Read the model definition and answer for the solid it produces. Units are mm, in the model's axes. Round coordinates to 2 decimals unless told otherwise and drop trailing zeros. Order: outer loops, then holes, each group sorted by start corner. A loop starts at its lowest first (then second) coordinate and runs counter-clockwise, first axis right, second up. Notation, with made-up numbers: (24.25, -1) -> (68.25, -1) arc R21 cw to (68.25, 31) -> close; hole circle Ø5 at (1, -21.75). An arc over 180 degrees is marked (long way). One line per item, written item: value. Start each with the question number.
1. Consider line 1 (X direction, y = 0.8, z = -5.5) (3 decimals); line 2 (X direction, y = 0.9, z = -1.75) (3 decimals). Determine where each line is inside the solid, lowest interval first.
2. A flat-ended cylindrical pin translates along its axis: pin 1 Ø3 at (x, z) = (-4, 3) entering from -Y. Find the tip coordinate at first contact, or state that the pin passes through.
3. Section B-B (x = 5) is taken. Give the vertices of the cut face in (y, z) (3 decimals).
4. Section C-C (y = 0.3) is taken. State how many separate pieces and enclosed holes the cut face has, then the cut area to 3 significant figures.
5. Section A-A (z = 3.5) is taken. Give the vertices of the cut face in (x, y) (3 decimals), then the cut area to 3 significant figures.
from build123d import *

# Parameters (mm, degrees)
SKETCH1_W           = 16.65
SKETCH1_H           = 16.65
SKETCH1_W_2         = 13.65
SKETCH1_H_2         = 13.65
SKETCH1_W_3         = 6.175
SKETCH1_H_3         = 1.3
SKETCH1_W_4         = 1.3
SKETCH1_H_4         = 6.175
BOSS_EXTRUDE1_DEPTH = 1
FILLET1_R           = 1.15


with BuildPart() as part:
    # Sketch1 → Boss-Extrude1 (new body)
    # profile 1 of 6: a face of its own
    with BuildSketch(Plane(origin=(0, 0, 0), x_dir=(1, 0, 0), z_dir=(0, 1, 0))):
        Rectangle(SKETCH1_W, SKETCH1_H)
        Rectangle(SKETCH1_W_2, SKETCH1_H_2, mode=Mode.SUBTRACT)
    # profile 2 of 6: a face of its own
    with BuildSketch(Plane(origin=(0, 0, 0), x_dir=(1, 0, 0), z_dir=(0, 1, 0))):
        with Locations((-3.7375, 0)):
            Rectangle(SKETCH1_W_3, SKETCH1_H_3)
    # profile 3 of 6: a face of its own
    with BuildSketch(Plane(origin=(0, 0, 0), x_dir=(1, 0, 0), z_dir=(0, 1, 0))):
        Rectangle(SKETCH1_W_4, SKETCH1_H_3)
    # profile 4 of 6: a face of its own
    with BuildSketch(Plane(origin=(0, 0, 0), x_dir=(1, 0, 0), z_dir=(0, 1, 0))):
        with Locations((0, -3.7375)):
            Rectangle(SKETCH1_W_4, SKETCH1_H_4)
    # profile 5 of 6: a face of its own
    with BuildSketch(Plane(origin=(0, 0, 0), x_dir=(1, 0, 0), z_dir=(0, 1, 0))):
        with Locations((3.7375, 0)):
            Rectangle(SKETCH1_W_3, SKETCH1_H_3)
    # profile 6 of 6: a face of its own
    with BuildSketch(Plane(origin=(0, 0, 0), x_dir=(1, 0, 0), z_dir=(0, 1, 0))):
        with Locations((0, 3.7375)):
            Rectangle(SKETCH1_W_4, SKETCH1_H_4)
    extrude(amount=BOSS_EXTRUDE1_DEPTH)

    # Fillet1
    fillet1_edges = [part.edges().sort_by_distance(p)[0] for p in [
        (-6.825, 0.5, 0.65),
        (-6.825, 0.5, 6.825),
        (-0.65, 0.5, 6.825),
        (-0.65, 0.5, 0.65),
        (-8.325, 0.5, 8.325),
        (-8.325, 0.5, -8.325),
        (8.325, 0.5, -8.325),
        (8.325, 0.5, 8.325),
        (-0.65, 0.5, -6.825),
        (-6.825, 0.5, -6.825),
        (-6.825, 0.5, -0.65),
        (-0.65, 0.5, -0.65),
        (0.65, 0.5, 6.825),
        (6.825, 0.5, 6.825),
        (6.825, 0.5, 0.65),
        (0.65, 0.5, 0.65),
        (6.825, 0.5, -0.65),
        (6.825, 0.5, -6.825),
        (0.65, 0.5, -6.825),
        (0.65, 0.5, -0.65),
    ]]
    fillet(fillet1_edges, radius=FILLET1_R)


solid = part.part
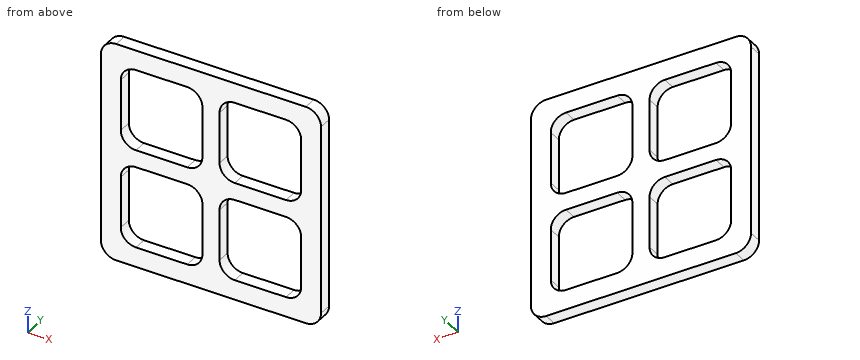
Answer:
1. line 1: -8.325 to -6.825, -0.65 to 0.65, 6.825 to 8.325
1. line 2: -8.325 to -6.824, -0.651 to 0.651, 6.824 to 8.325
2. pin 1: through
3. outline: (0, -8.325) -> (1, -8.325) -> (1, -6.825) -> (0, -6.825) -> close; (0, -0.65) -> (1, -0.65) -> (1, 0.65) -> (0, 0.65) -> close; (0, 6.825) -> (1, 6.825) -> (1, 8.325) -> (0, 8.325) -> close
4. separate pieces: 1
4. enclosed holes: 4
4. area: 128 mm^2
5. outline: (-8.325, 0) -> (-6.825, 0) -> (-6.825, 1) -> (-8.325, 1) -> close; (-0.65, 0) -> (0.65, 0) -> (0.65, 1) -> (-0.65, 1) -> close; (6.825, 0) -> (8.325, 0) -> (8.325, 1) -> (6.825, 1) -> close
5. area: 4.30 mm^2
